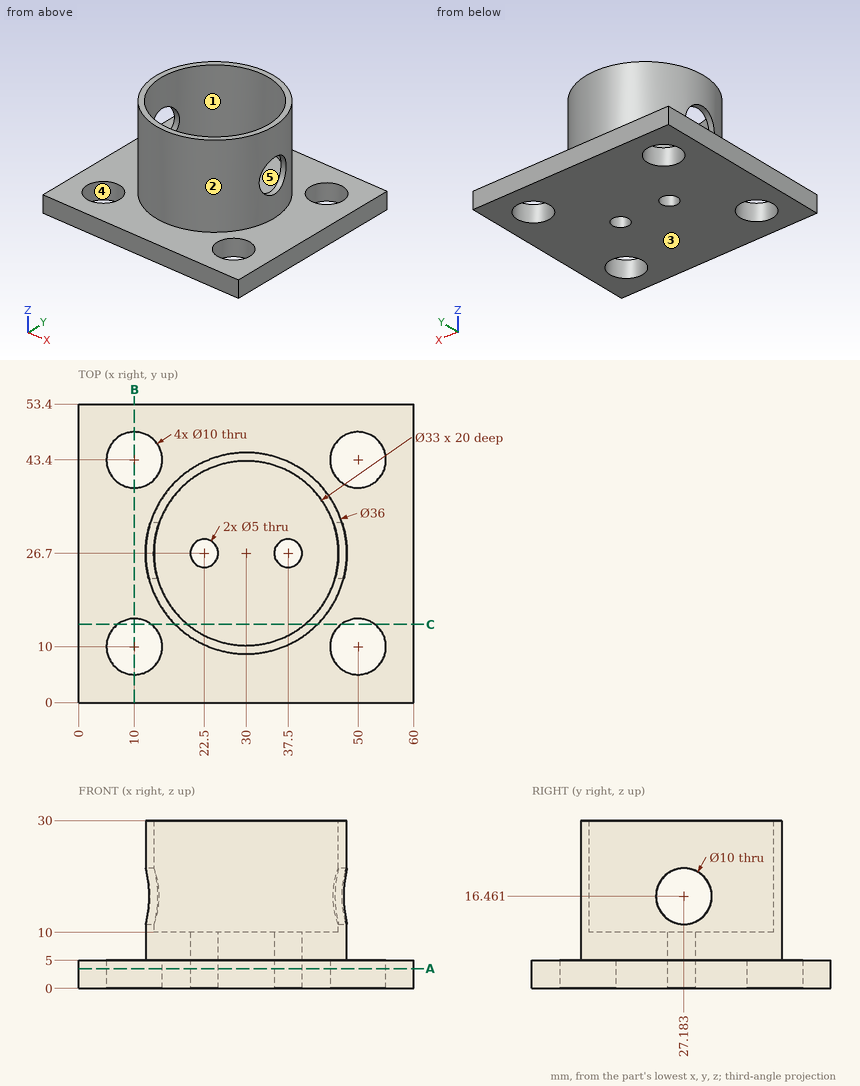
Job drawing, mm, ordinate dimensions from the low corner. One solid piece. A direction names the side the tool comes from. Give positions to 0.01 mm unless a question says otherwise; leave off trailing zeros. Loops run counter-clockwise (first coordinate to the right, second up) from the corner with the lowest first, then second, coordinate; pieces in that order, holes last. Notation, with made-up numbers: M -2,72 L 30,72 A18 cw 30,91 Z; hole C 46,41 d7. An arc over 180 degrees is marked long. Answer in a Markdown table with one row per item. Add a question column.
Item 1: Band-saw the part on C-C on y = 14. Give the cut face in (x, z) (1 decimal).
Item 2: Band-saw the part on B-B on x = 10. Give the cut face in (y, z), then the cut area to 3 significant figures.
Item 3: Tool access for the marked faces 4 and 5: list every direction of +Z, -Z, +X, -X, +Y, -Y with a clear straight run to the whole face (end or side of a thin tool).
Item 4: Probe probe 1 along Y at (x, z) = (10, 2.35); probe 2 along X at (y, z) = (43, 2) (1 decimal); probe 3 along Y at (x, z) = (30, 17). List the from-to ranges inside material, lowest first.
Item 5: Band-saw the part on A-A on z = 3.5. Give the cut face in (x, y), then the cut area to 3 significant figures.
Item 6: Drop flat-ended pins along their axis: P1, Ø12, axis at x = 38, z = 24.5, coming from the +Y side; P2, Ø10, axis at y = 17.5, z = 19, coming from the -X side; P3, Ø2, axis at x = 33.5, z = 16, coming from the +Y side (1 decimal). Give the stop position or say it passes through.
Item 7: Mould opens along X. For the marked faces 1, 2 and 3 say: +X half, -X half, draft (parallel to the pull), parting line (faces both ways), or undercut.
Reply:
| question | item | result |
|---|---|---|
| 1 | outline | M 0,0 L 7,0 L 7,5 L 0,5 Z; M 13,0 L 47,0 L 47,5 L 42.8,5 L 42.8,30 L 40.5,30 L 40.5,10 L 19.5,10 L 19.5,30 L 17.2,30 L 17.2,5 L 13,5 Z; M 53,0 L 60,0 L 60,5 L 53,5 Z |
| 2 | outline | M 0,0 L 5,0 L 5,5 L 0,5 Z; M 15,0 L 38.4,0 L 38.4,5 L 15,5 Z; M 48.4,0 L 53.4,0 L 53.4,5 L 48.4,5 Z |
| 2 | area | 167 mm^2 |
| 3 | face 4 | +Z, -Z |
| 3 | face 5 | +Z |
| 4 | probe 1 | y = 0 to 5, 15 to 38.4, 48.4 to 53.4 |
| 4 | probe 2 | x = 0 to 5, 15 to 45, 55 to 60 |
| 4 | probe 3 | y = 8.7 to 10.2, 43.2 to 44.7 |
| 5 | outline | M 0,0 L 60,0 L 60,53.4 L 0,53.4 Z; hole C 10,10 d10; hole C 10,43.4 d10; hole C 22.5,26.7 d5; hole C 37.5,26.7 d5; hole C 50,10 d10; hole C 50,43.4 d10 |
| 5 | area | 2,850 mm^2 |
| 6 | P1 | stops at y = 44.59 |
| 6 | P2 | stops at x = 12.5 |
| 6 | P3 | stops at y = 44.5 |
| 7 | face 1 | undercut |
| 7 | face 2 | parting line |
| 7 | face 3 | draft |
